Geometry: see drawing. Coordinates: mm, zero at the bounding-box minimum. A direction names the side the tool comes from. Give positions to 0.01 mm unless a question says otherwise; leave off trailing zeros. Loops run counter-clockwise (first coordinate to the right, second up) from the corner with the lowest first, then second, coordinate; pieces in that order, holes last. Notation, with made-up numbers: (64, 81) -> (106, 81) arc R25 ccw to (106, 110) -> close; hole circle Ø9 at (-28.5, 80). An arc over 180 degrees is marked (long way). Answer in a Markdown table with one row per item. Add a question column.
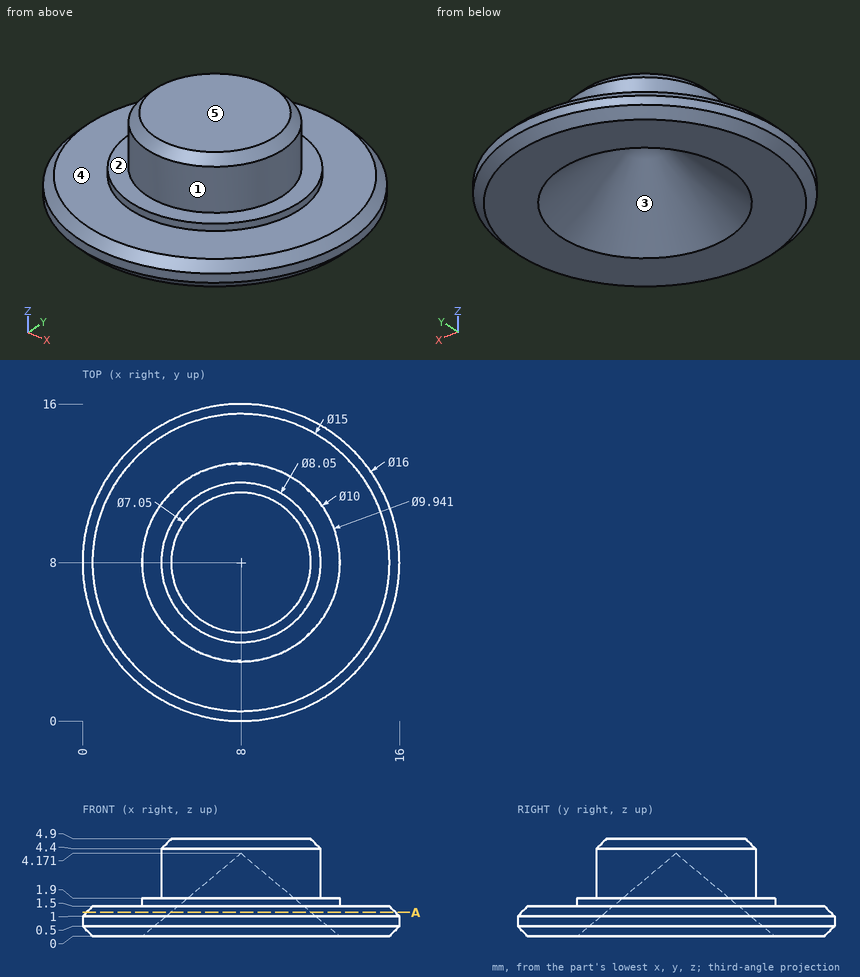
1) Pin query (flat end, axial travel): pin 1 (2 mm diameter, centred on y = 2.5, z = 2, fed in from +X) (1 decimal); pin 2 (6 mm diameter, centred on x = 8, y = 6.5, fed in from -Z) (1 decimal); pin 3 (2 mm diameter, centred on y = 9.5, z = 4.5, fed in from +X). Return the tip coordinate at first contact, or that it passes through.
2) Material intervals for line 1 along Z through (x, y) = (5, 14.75); line 2 along X through (y, z) = (7.25, 0.75) (1 decimal); line 3 along Y through (x, z) = (7, 0.85) (1 decimal), sorted ascending.
3) Reachability of the marked faces 4 and 5 from +Z, -Z, +X, -X, +Y, -Y: full face, straight path, thin tool, end or side. Return the list, or none.
4) Pull-direction query (Y, two-part tool) for the marked faces 1, 2 and 3; classes: +Y half, -Y half, draft (parallel to the pull), parting line (faces both ways), or undercut.
5) Section A-A on z = 1.2. Output: boundary loops of the cut face in (x, y), and give its area (3 significant figures).
Working result:
| question | item | result |
|---|---|---|
| 1 | pin 1 | stops at x = 14.1 |
| 1 | pin 2 | stops at z = 0.4 |
| 1 | pin 3 | stops at x = 11.99 |
| 2 | line 1 | z = 0 to 1.5 |
| 2 | line 2 | x = 0 to 4, 12 to 16 |
| 2 | line 3 | y = 0.1 to 4.2, 11.8 to 15.9 |
| 3 | face 4 | +Z |
| 3 | face 5 | +Z, +X, -X, +Y, -Y |
| 4 | face 1 | parting line |
| 4 | face 2 | draft |
| 4 | face 3 | undercut |
| 5 | outline | circle Ø15.6 at (8, 8); hole circle Ø7.08 at (8, 8) |
| 5 | area | 152 mm2 |
